Autodesk Fusion 360 part; units mm, degrees
sketch "Sketch1" plane through (0, 0, 0) normal (0, 0, 1) x (1, 0, 0)
  line L0 (0, 0) -> (171, 0)
  line L1 (171, 0) -> (171, 80)
  line L2 (171, 80) -> (0, 80)
  line L3 (0, 80) -> (0, 0)
  dimension "d1" = 171
  dimension "d2" = 80
extrude "Extrude1" add sketch "Sketch1" along normal blind 59
sketch "Sketch2" plane through (0, 0, 59) normal (0, 0, 1) x (-1, 0, 0)
  line L0 (0, -80) -> (0, 0)
  line L1 (0, 0) -> (-171, 0)
  line L2 (-171, 0) -> (-171, -80)
  line L3 (-171, -80) -> (0, -80)
  line L4 (-166, -5) -> (-88, -5)
  line L5 (-88, -5) -> (-88, -75)
  line L6 (-88, -75) -> (-166, -75)
  line L7 (-166, -75) -> (-166, -5)
  line L8 (-85.5, 0) -> (-85.5, -80)
  line L9 (-5, -5) -> (-83, -5)
  line L10 (-5, -75) -> (-5, -5)
  line L11 (-83, -5) -> (-83, -75)
  line L12 (-83, -75) -> (-5, -75)
  dimension "d5" = 85.5
  dimension "d6" = 70
  dimension "d8" = 5
  dimension "d9" = 5
  dimension "d10" = 2.5
  dimension "d11" = 5
extrude "Extrude2" cut sketch "Sketch2" against normal blind 10 contours L4 L5 L6 L7 | L9 L10 L11 L12
extrude "Extrude3" cut 2 faces at (57, 28.3333, 49) (140, 28.3333, 49) along direction (0, 0, -1) blind 10
sketch "Sketch3" plane through (0, 0, 59) normal (0, 0, 1) x (-1, 0, 0)
  line L0 (-88, -5) -> (-88, -75)
  line L1 (-88, -75) -> (-166, -75)
  line L2 (-166, -75) -> (-166, -5)
  line L3 (-166, -5) -> (-88, -5)
  line L4 (-5, -5) -> (-5, -75)
  line L5 (-5, -75) -> (-83, -75)
  line L6 (-83, -75) -> (-83, -5)
  line L7 (-83, -5) -> (-5, -5)
  line L8 (0, -80) -> (0, 0)
  line L9 (0, 0) -> (-171, 0)
  line L10 (-171, 0) -> (-171, -80)
  line L11 (-171, -80) -> (0, -80)
  circle A0 centre (-85.5, -65) radius 10
  line L12 (-85.5, 0) -> (-85.5, -80)
  line L13 (-83, -75) -> (-5, -75)
  circle A1 centre (-85.5, -65) radius 15
  dimension "d16" = 20
  dimension "d17" = 10
  dimension "d18" = 30
extrude "Extrude4" add sketch "Sketch3" against normal blind 20 contours L0 L1 A0 A1 | L5 L6 A0 L13 A1
extrude "Extrude5" cut sketch "Sketch3" against normal blind 20 contours L0 A0 L12 | L6 A0 L12
sketch "Sketch4" plane through (0, 0, 0) normal (0, -1, 0) x (1, 0, 0)
  line L0 (0, 0) -> (171, 0)
  line L1 (171, 0) -> (171, 59)
  line L2 (171, 59) -> (0, 59)
  line L3 (0, 59) -> (0, 0)
  line L4 (0, 0) -> (171, 0)
  line L5 (171, 0) -> (171, 30)
  line L6 (171, 30) -> (0, 30)
  line L7 (0, 30) -> (0, 0)
  dimension "d23" = 30
extrude "Extrude6" cut sketch "Sketch4" against normal blind 80 contours L0 L1 L3 L4 L5 L6 L7
sketch "Sketch5" plane through (0, 0, 30) normal (0, 0, -1) x (1, 0, 0)
  line L0 (171, 0) -> (0, 0)
  line L1 (0, 0) -> (0, -80)
  line L2 (0, -80) -> (171, -80)
  line L3 (171, -80) -> (171, 0)
  line L4 (166, -75) -> (5, -75)
  line L5 (5, -75) -> (5, -5)
  line L6 (5, -5) -> (166, -5)
  line L7 (166, -5) -> (166, -75)
  point P0 (166, -75)
  point P1 (5, -5)
extrude "Extrude7" cut sketch "Sketch5" against normal blind 3
Work out the finished part from the listing and answer in its coordinate system (mm). A direction names the side the tool comes from. Round coordinates to 2 decimals unless told otherwise and drop trailing zeros. Loops run counter-clockwise (first coordinate to the right, second up) from the corner with the lowest first, then second, coordinate; pieces in that order, holes last. Notation, with made-up numbers: M 17,-29 L 30,-29 A10 cw 30,-24 Z; hole C -37.75,-0.75 d9. An arc over 180 degrees is marked long. One line per question, with ' | ' between items. Start each with the question number.
(1) A cutting plane is placed at D-D on y = 34. Write down the section's boundary in (x, z).
(2) For a pull along X with two mould halves and no side action, classify faces 4 (the face through (166, 40, 31)), 5 (the face through (84, 5, 31)), 6 (the face through (5, 40, 31)), 7 (the face through (79.5, 57, 49.1)) as released by +X, released by -X, zero draft, split by the parting line, or undercut.
(3) A cutting plane is placed at C-C on z = 45.25. Write down the section's boundary in (x, y), plus the area to 3 significant figures.
(4) A cutting plane is placed at A-A on y = 65. Write down the section's boundary in (x, z), plus the area to 3 significant figures.
(5) A cutting plane is placed at B-B on x = 126. Write down the section's boundary in (y, z).
(6) Flat-ended cylindrical pins translate along their axes: pin 1 Ø1 at (x, y) = (51.5, 17) entering from +Z; pin 2 Ø1.5 at (x, z) = (71.5, 31) entering from -Y; pin 3 Ø1.5 at (y, z) = (45.5, 31) entering from +X. Find the tip coordinate at first contact, or state that the pin passes through.
(7) A tool of negligible diameter and unlimited length cuts with its end or side. For faces 1 (the face through (87, 75, 31)), 2 (the face through (85, 40, 59)), 3 (the face through (131, 75, 49)), from which of +Z, -Z, +X, -X, +Y, -Y can it reach the whole face along a straight path? Write none if from no direction.
(8) Find the intervals of material crossed by line 1 (X direction, y = 65, z = 46.5); line 2 (X direction, y = 34.5, z = 39.25); line 3 (Y direction, x = 85, z = 48), in increasing order.
Geometry check:
1) outline: M 0,33 L 5,33 L 5,30 L 166,30 L 166,33 L 171,33 L 171,59 L 166,59 L 166,39 L 88,39 L 88,59 L 83,59 L 83,39 L 5,39 L 5,59 L 0,59 Z
2) face 4: released by +X | face 5: zero draft | face 6: released by -X | face 7: undercut
3) outline: M 0,0 L 171,0 L 171,80 L 0,80 Z; hole M 5,5 L 83,5 L 83,50.21 A15 cw 74.32,75 L 5,75 Z; hole C 85.5,65 d20; hole M 88,5 L 166,5 L 166,75 L 96.68,75 A15 cw 88,50.21 Z | area: 2,950 mm²
4) outline: M 0,33 L 5,33 L 5,30 L 166,30 L 166,33 L 171,33 L 171,59 L 166,59 L 166,39 L 100.5,39 L 100.5,59 L 95.5,59 L 95.5,39 L 75.5,39 L 75.5,59 L 70.5,59 L 70.5,39 L 5,39 L 5,59 L 0,59 Z | area: 1,910 mm²
5) outline: M 0,33 L 5,33 L 5,30 L 75,30 L 75,33 L 80,33 L 80,59 L 75,59 L 75,39 L 5,39 L 5,59 L 0,59 Z
6) pin 1: stops at z = 39 | pin 2: stops at y = 5 | pin 3: stops at x = 166
7) face 1: -Z, +X, -X, +Y | face 2: +Z, +X, -X, +Y, -Y | face 3: +Z
8) line 1: x = 0 to 5, 70.5 to 75.5, 95.5 to 100.5, 166 to 171 | line 2: x = 0 to 5, 83 to 88, 166 to 171 | line 3: y = 0 to 55.01, 74.99 to 80
